The listing builds one solid part. Answer for the finished solid, in the listing's coordinates (mm). Face numbers are marked on the shaded views. A direction names the side the tool comes from. Coordinates: 2 decimals unless noted, no trailing zeros. Loops run counter-clockwise (first coordinate to the right, second up) from the corner with the lowest first, then second, coordinate; pieces in that order, holes last. Notation, with made-up numbers: M -37.75,-16.5 L -15.75,-16.5 A34 ccw -15.75,22.5 Z; hole C -2.75,83 d6. An arc over 180 degrees is marked long. Answer as a JSON object with one key per item and string values. Group by question number.
1. A cutting plane is placed at D-D on z = 1. Give the vertices of the cut face in (x, y), and give its area (3 significant figures).
2. Straight lines are drawn through the part: L1, parallel to X at y = 22.75, z = 4; L2, parallel to X at y = 22, z = 2; L3, parallel to X at y = 45, z = 1. For each, find the intervals that lie inside material, in ascending order.
3. A cutting plane is placed at C-C on x = -27. Give the vertices of the cut face in (y, z).
4. A cutting plane is placed at B-B on y = 40. Give the vertices of the cut face in (x, z), and give its area (3 significant figures).
5. For the marked faces 1, 2 and 3, determine the directions among +Z, -Z, +X, -X, +Y, -Y from which every point of the face is accessible in a straight line to the end or side of a thin tool.
6. Determine the mould class of the marked faces 4, 5 and 6 for opening direction X: released by +X, released by -X, zero draft, split by the parting line, or undercut.
7. Given pin 1 (1.5 mm diameter, centred on y = 30.5, z = 7, fed in from -X); pin 2 (1 mm diameter, centred on x = 1.5, z = 6, fed in from +Y), each flat-ended and moving along its own axis, determine where each tip first touches the part or whether it passes through.
8. A cutting plane is placed at A-A on z = 3. Give the vertices of the cut face in (x, y), and give its area (3 significant figures).
from build123d import *

# Parameters (mm, degrees)
SKETCH2_R           = 4
BOSS_EXTRUDE1_DEPTH = 8
SKETCH3_R           = 2.5
CUT_EXTRUDE1_DEPTH  = 6.65


with BuildPart() as part:
    # Sketch2 → Boss-Extrude1 (new body)
    with BuildSketch(Plane.XY):
        Polygon((-32.285858586, 18.527272727), (-32.285858586, 25.177272727), (-20.285858586, 25.177272727), (-20.285858586, 50.177272727), (-2.285858586, 50.177272727), (-2.285858586, 25.177272727), (9.714141414, 25.177272727), (9.714141414, 18.527272727), align=None)
        with Locations((-11.285858586, 38.777272727)):
            Circle(SKETCH2_R, mode=Mode.SUBTRACT)
    extrude(amount=BOSS_EXTRUDE1_DEPTH)

    # Sketch3 → Cut-Extrude1 (cut)
    with BuildSketch(Plane(origin=(0, 25.177272727, 0), x_dir=(1, 0, 0), z_dir=(0, 1, 0))):
        with Locations(Location((-26.285858586, -4, 0), (0, 0, 270))):
            Circle(SKETCH3_R)
        with Locations(Location((3.45668569, -4, 0), (0, 0, 270))):
            Circle(SKETCH3_R)
    extrude(amount=-CUT_EXTRUDE1_DEPTH, mode=Mode.SUBTRACT)


solid = part.part
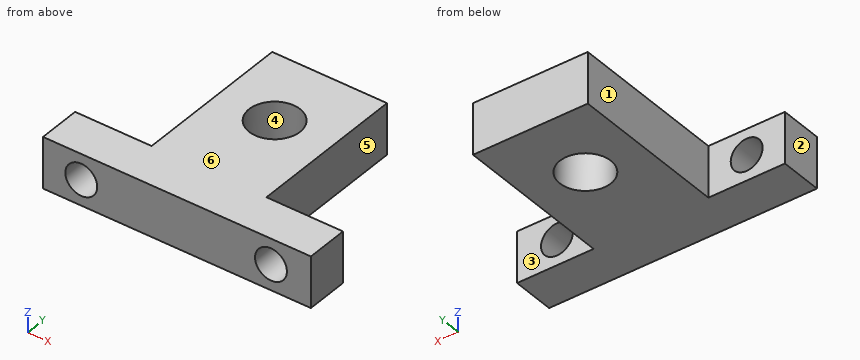
From the geometry:
{
 "1": {"outline": "M -32.29,18.53 L 9.71,18.53 L 9.71,25.18 L -2.29,25.18 L -2.29,50.18 L -20.29,50.18 L -20.29,25.18 L -32.29,25.18 Z; hole C -11.29,38.78 d8", "area": "679 mm²"},
 "2": {"L1": "x = -32.29 to -28.79, -23.79 to 0.96, 5.96 to 9.71", "L2": "x = -32.29 to -27.79, -24.79 to 1.96, 4.96 to 9.71", "L3": "x = -20.29 to -2.29"},
 "3": {"outline": "M 18.53,0 L 25.18,0 L 25.18,1.6 L 18.53,1.6 Z; M 18.53,6.4 L 25.18,6.4 L 25.18,8 L 18.53,8 Z"},
 "4": {"outline": "M -20.29,0 L -15.09,0 L -15.09,8 L -20.29,8 Z; M -7.48,0 L -2.29,0 L -2.29,8 L -7.48,8 Z", "area": "83.1 mm²"},
 "5": {"face 1": "+Z, -Z, -X, +Y", "face 2": "+Z, -Z, -X, +Y, -Y", "face 3": "+Z, -Z, +X, +Y"},
 "6": {"face 4": "undercut", "face 5": "released by +X", "face 6": "zero draft"},
 "7": {"pin 1": "stops at x = -20.29", "pin 2": "stops at y = 25.18"},
 "8": {"outline": "M -32.29,18.53 L -28.58,18.53 L -28.58,25.18 L -32.29,25.18 Z; M -23.99,18.53 L 1.17,18.53 L 1.17,25.18 L -2.29,25.18 L -2.29,50.18 L -20.29,50.18 L -20.29,25.18 L -23.99,25.18 Z; M 5.75,18.53 L 9.71,18.53 L 9.71,25.18 L 5.75,25.18 Z; hole C -11.29,38.78 d8", "area": "618 mm²"}
}
